Build history of the part. All positions in model axes, mm. A direction names the side the tool comes from. Round coordinates to 2 decimals unless told otherwise and drop trailing zeros. Write each loop counter-clockwise with the first axis right and the second up, starting at its lowest first coordinate (ties: lowest second). Pieces come first, ordered by that corner, then holes. Notation, with made-up numbers: (-35, 67.25) -> (-4, 67.25) arc R18 cw to (-4, 102.25) -> close; hole circle Ø2 at (13.25, -8). An arc over 180 degrees is marked (long way). One line per question, with ' | ' between items.
from build123d import *

# Parameters (mm, degrees)
F1_DEPTH = 127


with BuildPart() as f1:
    # F0 (on Front) → F1 (new body)
    with BuildSketch(Plane.XZ):
        with BuildLine():
            ThreePointArc((63.5, 57.15), (61.640128, 61.640128), (57.15, 63.5))
            Line((57.15, 63.5), (-57.15, 63.5))
            ThreePointArc((-57.15, 63.5), (-61.640128, 61.640128), (-63.5, 57.15))
            Line((-63.5, 57.15), (-63.5, -57.15))
            ThreePointArc((-63.5, -57.15), (-61.640128, -61.640128), (-57.15, -63.5))
            Line((-57.15, -63.5), (57.15, -63.5))
            ThreePointArc((57.15, -63.5), (61.640128, -61.640128), (63.5, -57.15))
            Line((63.5, -57.15), (63.5, 57.15))
        make_face()
        with BuildLine():
            Line((55.290128, -61.640128), (-55.290128, -61.640128))
            ThreePointArc((-55.290128, -61.640128), (-59.780256, -59.780256), (-61.640128, -55.290128))
            Line((-61.640128, -55.290128), (-61.640128, -6.35))
            ThreePointArc((-61.640128, -6.35), (-59.780256, -1.859872), (-55.290128, 0))
            Line((-55.290128, 0), (55.290128, 0))
            ThreePointArc((55.290128, 0), (59.780256, -1.859872), (61.640128, -6.35))
            Line((61.640128, -6.35), (61.640128, -55.290128))
            ThreePointArc((61.640128, -55.290128), (59.780256, -59.780256), (55.290128, -61.640128))
        make_face(mode=Mode.SUBTRACT)
        with BuildLine():
            ThreePointArc((-55.879999, 52.781393), (-54.020127, 57.271521), (-49.529999, 59.131393))
            Line((-49.529999, 59.131393), (52.070001, 59.131393))
            ThreePointArc((52.070001, 59.131393), (56.56013, 57.271521), (58.420001, 52.781393))
            Line((58.420001, 52.781393), (58.420001, 27.381393))
            ThreePointArc((58.420001, 27.381393), (56.56013, 22.891265), (52.070001, 21.031393))
            Line((52.070001, 21.031393), (-49.529999, 21.031393))
            ThreePointArc((-49.529999, 21.031393), (-54.020127, 22.891265), (-55.879999, 27.381393))
            Line((-55.879999, 27.381393), (-55.879999, 52.781393))
        make_face(mode=Mode.SUBTRACT)
    extrude(amount=F1_DEPTH)


solid = f1.part
(1) Slice it at D-D (z = -35). Write the cut outline in (x, y), then the cut area to 3 significant figures.
Calculated:
outline: (-63.5, -127) -> (-61.64, -127) -> (-61.64, 0) -> (-63.5, 0) -> close; (61.64, -127) -> (63.5, -127) -> (63.5, 0) -> (61.64, 0) -> close | area: 472 mm2
(2) Wall check: line 1 (Z direction, x = -30.5, y = -113); line 2 (X direction, y = -99, z = 51); line 3 (X direction, y = -102, z = -32). Give the ranges that are in metal, low to high. Write a range as from..to.
Calculated:
line 1: -63.5..-61.64, 0..21.03, 59.13..63.5 | line 2: -63.5..-55.88, 58.42..63.5 | line 3: -63.5..-61.64, 61.64..63.5
(3) Slice it at C-C (z = 48.5). Write the cut outline in (x, y).
Calculated:
outline: (-63.5, -127) -> (-55.88, -127) -> (-55.88, 0) -> (-63.5, 0) -> close; (58.42, -127) -> (63.5, -127) -> (63.5, 0) -> (58.42, 0) -> close
(4) Slice it at B-B (y = -16.5). Write the cut outline in (x, z).
Calculated:
outline: (-63.5, -57.15) arc R6.35 ccw to (-57.15, -63.5) -> (57.15, -63.5) arc R6.35 ccw to (63.5, -57.15) -> (63.5, 57.15) arc R6.35 ccw to (57.15, 63.5) -> (-57.15, 63.5) arc R6.35 ccw to (-63.5, 57.15) -> close; hole (-61.64, -55.29) arc R6.35 ccw to (-55.29, -61.64) -> (55.29, -61.64) arc R6.35 ccw to (61.64, -55.29) -> (61.64, -6.35) arc R6.35 ccw to (55.29, 0) -> (-55.29, 0) arc R6.35 ccw to (-61.64, -6.35) -> close; hole (-55.88, 27.38) arc R6.35 ccw to (-49.53, 21.03) -> (52.07, 21.03) arc R6.35 ccw to (58.42, 27.38) -> (58.42, 52.78) arc R6.35 ccw to (52.07, 59.13) -> (-49.53, 59.13) arc R6.35 ccw to (-55.88, 52.78) -> close
(5) Slice it at A-A (x = 32). Write the cut outline in (y, z).
Calculated:
outline: (-127, -63.5) -> (0, -63.5) -> (0, -61.64) -> (-127, -61.64) -> close; (-127, 0) -> (0, 0) -> (0, 21.03) -> (-127, 21.03) -> close; (-127, 59.13) -> (0, 59.13) -> (0, 63.5) -> (-127, 63.5) -> close
(6) 3-axis set-ups, long thin cutter, end or side, ignore diameter. For faces 4 (the flat face through (61.64, -63, -30)), 5 (the flat face through (-63.5, -63, 1)): which of +Z, -Z, +X, -X, +Y, -Y reach the whole face in a straight line?
Calculated:
face 4: +Y, -Y | face 5: +Z, -Z, -X, +Y, -Y
(7) Mould opens along Z. For faces 1 (the flat face through (63.5, -63, -1)), 2 (the cylindrical face through (-59.83, -62.61, -1.91)), 3 (the cylindrical face through (61.59, -62.61, -61.69)) say: pulls with the +Z half, pulls with the -Z half, needs draft (parallel to the pull), parting line crosses it, or undercut.
Calculated:
face 1: needs draft | face 2: undercut | face 3: pulls with the -Z half
